from build123d import *

# Parameters (mm, degrees)
BOSS_EXTRUDE1_DEPTH        = 3
BOSS_EXTRUDE1_DEPTH_BACK   = 10
SKETCH1_R                  = 10
SKETCH4_R                  = 1.5
HOLE_DEPTH                 = 20.973741561
HOLECIR_COUNT              = 5
SKETCH6_W                  = 7
SKETCH6_H                  = 7
BEARINGHOLE_DEPTH          = 2.5
SKETCH7_R                  = 2.05
SHAFTHOLE_DEPTH            = 17.248076982
F_3_1_3_1_DIAMETER_HOLE1_D = 3.1
FILLET2_R                  = 3
SKETCH11_R                 = 10
CUT_EXTRUDE1_DEPTH         = 10


with BuildPart() as part:
    # Sketch1 → Boss-Extrude1 (new, two sides: drawn at the far end of the back side and taken through both)
    with BuildSketch(Plane(origin=(0, 0, 0), x_dir=(1, 0, 0), z_dir=(0, 1, 0)).offset(-BOSS_EXTRUDE1_DEPTH_BACK)):
        with Locations(Location((0, 0, 0), (0, 0, 270))):
            Circle(SKETCH1_R)
    extrude(amount=BOSS_EXTRUDE1_DEPTH + BOSS_EXTRUDE1_DEPTH_BACK)

    # Sketch4 → hole (cut, through all)
    with BuildSketch(Plane(origin=(-3.352872105, -1.093066116, 1.887711608), x_dir=(-0.4486862613641547, -0.14627571033740308, -0.8816371449912632), z_dir=(0.8382180262940947, 0.2732665289126682, -0.47192790187872385))):
        with Locations(Location((0, 0, 0), (0, 0, 8.746528197))):
            Circle(SKETCH4_R)
    hole = extrude(amount=-HOLE_DEPTH, mode=Mode.SUBTRACT)

    # holecir: hole ×5 about axis
    holecir_axis = Axis((0, 0, 0), (0, 1, 0))
    for i in range(1, HOLECIR_COUNT):
        add(hole.rotate(holecir_axis, i * 360 / HOLECIR_COUNT), mode=Mode.SUBTRACT)

    # Sketch6 → bearinghole (cut)
    with BuildSketch(Plane(origin=(0, -5, 0), x_dir=(-1, 0, 0), z_dir=(0, -1, 0))):
        Rectangle(SKETCH6_W, SKETCH6_H)
    extrude(amount=BEARINGHOLE_DEPTH, mode=Mode.SUBTRACT)

    # Sketch7 → shafthole (cut, through all)
    with BuildSketch(Plane(origin=(0, -5, 0), x_dir=(-1, 0, 0), z_dir=(0, -1, 0))):
        with Locations(Location((0, 0, 0), (0, 0, 270))):
            Circle(SKETCH7_R)
    extrude(amount=SHAFTHOLE_DEPTH, mode=Mode.SUBTRACT)

    # Ø3.1 (3.1) Diameter Hole1 (through all)
    with Locations(Plane(origin=(0, 3, 0), x_dir=(1, 0, 0), z_dir=(0, 1, 0))):
        with Locations((-1.282558474, 6.372208703), (4.783101903, -4.401356176)):
            Hole(F_3_1_3_1_DIAMETER_HOLE1_D / 2)

    # Fillet2
    # the kernel refuses this fillet: 3 mm, written as the material it takes off along each edge
    with BuildSketch(Plane(origin=(0, 3, 0), x_dir=(0, 0, 1), z_dir=(-1, 0, 0))) as fillet2_piece_1:
        with BuildLine():
            CenterArc((10 - FILLET2_R, -FILLET2_R), FILLET2_R, 0, 90)
            Line((10 - FILLET2_R, 0), (10, 0))
            Line((10, 0), (10, -FILLET2_R))
        make_face()
    revolve(axis=Axis((0, 3, 0), (0, 1, 0)), mode=Mode.SUBTRACT)
    with BuildSketch(Plane(origin=(0, -10, 0), x_dir=(0, 0, 1), z_dir=(-1, 0, 0))) as fillet2_piece_2:
        with BuildLine():
            CenterArc((10 - FILLET2_R, FILLET2_R), FILLET2_R, 270, 90)
            Line((10 - FILLET2_R, 0), (10, 0))
            Line((10, 0), (10, FILLET2_R))
        make_face()
    revolve(axis=Axis((0, -10, 0), (0, 1, 0)), mode=Mode.SUBTRACT)

    # Sketch11 → Cut-Extrude1 (cut)
    with BuildSketch(Plane(origin=(0, -6.25, 0), x_dir=(-1, 0, 0), z_dir=(0, -1, 0))):
        with Locations(Location((0, 0, 0), (0, 0, 270))):
            Circle(SKETCH11_R)
    extrude(amount=-CUT_EXTRUDE1_DEPTH, mode=Mode.SUBTRACT)


solid = part.part
The model under review builds one solid part; all positions refer to its coordinate system, in mm. A direction names the side the tool comes from. Coordinates: 2 decimals unless noted, no trailing zeros. Loops run counter-clockwise (first coordinate to the right, second up) from the corner with the lowest first, then second, coordinate; pieces in that order, holes last. Notation, with made-up numbers: (51.25, 41) -> (57.25, 41) arc R29 ccw to (57.25, 71) -> close; hole circle Ø11 at (-6.5, 2). An arc over 180 degrees is marked (long way). Use a Markdown table: item, result. Add a question column.
1. To check wall thickness, follow line 1 (Y direction, x = 2.75, z = -0.25); line 2 (X direction, y = -7.5, z = -6.5); line 3 (X direction, y = -6.8, z = -5). State the ranges of each line that lie inside material, in increasing order.
2. Draft analysis for pull direction X (two halves, no side actions). For faces 3 (the face through (0, -7, 3.5)), 4 (the face through (0, -6.25, 4)), 5 (the face through (3.305, -8.151, 3.936)), 6 (the face through (-9.76, -6.63, -2.17)), state which applies: pulls with the +X half, pulls with the -X half, needs draft (parallel to the pull), parting line crosses it, or undercut.
3. Add section C-C on y = -9.1. Write out the cut boundary in (x, z).
4. Add section B-B on y = -6.5. Write out the cut boundary in (x, z).
5. Machinability: for faces 1 (the face through (0, -7, -3.5)), 2 (the face through (-2.033, -8.732, -0.267)), which of the approach directions +Z, -Z, +X, -X, +Y, -Y give a long, thin tool a straight path to every point of the face, cutting with its end or side? Answer none if there is none.
6. Clearance check with flat-ended pins moving along their axes: pin 1 Ø2 at (y, z) = (-8, 7) entering from -X; pin 2 Ø1 at (x, y) = (3, -9) entering from -Z; pin 3 Ø1.9 at (x, z) = (4.78, 4.4) entering from +Y; pin 4 Ø1 at (x, y) = (3.5, -7) entering from +Z. State where each tip first meets the part, or that it passes through.
7. Add section A-A on z = 0. Write out the cut boundary in (x, y), plus the area to 3 significant figures.
Returned:
| question | item | result |
|---|---|---|
| 1 | line 1 | y = -10 to -7.5 |
| 1 | line 2 | x = -7.54 to -2.83, 0.26 to 7.54 |
| 1 | line 3 | x = -8.66 to -2, -0.56 to 8.66 |
| 2 | face 3 | undercut |
| 2 | face 4 | needs draft |
| 2 | face 5 | undercut |
| 2 | face 6 | parting line crosses it |
| 3 | outline | circle Ø18.28 at (0, 0); hole circle Ø3.1 at (-1.28, -6.37); hole circle Ø4.1 at (0, 0); hole circle Ø3.1 at (4.78, 4.4) |
| 4 | outline | circle Ø20 at (0, 0); hole (-3.5, -3.5) -> (3.5, -3.5) -> (3.5, 3.5) -> (-3.5, 3.5) -> close; hole circle Ø3.1 at (-1.28, -6.37); hole circle Ø3.1 at (4.78, 4.4) |
| 5 | face 1 | +Y |
| 5 | face 2 | +Y, -Y |
| 6 | pin 1 | stops at x = -7.86 |
| 6 | pin 2 | stops at z = -9.16 |
| 6 | pin 3 | passes through |
| 6 | pin 4 | stops at z = 9.54 |
| 7 | outline | (-10, -7) arc R3 ccw to (-7, -10) -> (-2.05, -10) -> (-2.05, -7.5) -> (-3.5, -7.5) -> (-3.5, -6.25) -> (-10, -6.25) -> close; (2.05, -10) -> (7, -10) arc R3 ccw to (10, -7) -> (10, -6.25) -> (3.5, -6.25) -> (3.5, -7.5) -> (2.05, -7.5) -> close |
| 7 | area | 52.1 mm² |
